Autodesk Inventor part; units mm, degrees
ref_plane "YZ Plane" through (0, 0, 0) normal (1, 0, 0) x (0, 1, 0)
ref_plane "XZ Plane" through (0, 0, 0) normal (0, 1, 0) x (-1, 0, 0)
ref_plane "XY Plane" through (0, 0, 0) normal (0, 0, 1) x (1, 0, 0)
sketch "Sketch1" plane through (0, 0, 0) normal (0, 0, 1) x (1, 0, 0)
  circle A0 centre (0, 0) radius 161.1083
  line L0 (4.75, 161.0382) -> (4.75, -161.0382)
  line L1 (-4.75, -161.0382) -> (-4.75, 161.0382)
  line L2 (0, 0) -> (0, 161.1083) construction
  line L3 (23.8125, 79.375) -> (23.8125, 47.625)
  line L4 (23.8125, 47.625) -> (51.3088, 63.5)
  line L5 (51.3088, 63.5) -> (23.8125, 79.375)
  line L6 (23.8125, 111.125) -> (23.8125, 79.375)
  line L7 (23.8125, 79.375) -> (51.3088, 95.25)
  line L8 (51.3088, 95.25) -> (23.8125, 111.125)
  line L9 (23.8125, 47.625) -> (23.8125, 15.875)
  line L10 (23.8125, 15.875) -> (51.3088, 31.75)
  line L11 (51.3088, 31.75) -> (23.8125, 47.625)
  line L12 (23.8125, 15.875) -> (23.8125, -15.875)
  line L13 (23.8125, -15.875) -> (51.3088, 0)
  line L14 (51.3088, 0) -> (23.8125, 15.875)
  line L15 (23.8125, -15.875) -> (23.8125, -47.625)
  line L16 (23.8125, -47.625) -> (51.3088, -31.75)
  line L17 (51.3088, -31.75) -> (23.8125, -15.875)
  line L18 (23.8125, -47.625) -> (23.8125, -79.375)
  line L19 (23.8125, -79.375) -> (51.3088, -63.5)
  line L20 (51.3088, -63.5) -> (23.8125, -47.625)
  line L21 (23.8125, -79.375) -> (23.8125, -111.125)
  line L22 (23.8125, -111.125) -> (51.3088, -95.25)
  line L23 (51.3088, -95.25) -> (23.8125, -79.375)
  line L24 (51.3088, 95.25) -> (78.8051, 79.375)
  line L25 (78.8051, 79.375) -> (51.3088, 63.5)
  line L26 (51.3088, 63.5) -> (78.8051, 47.625)
  line L27 (78.8051, 47.625) -> (51.3088, 31.75)
  line L28 (51.3088, 31.75) -> (78.8051, 15.875)
  line L29 (78.8051, 15.875) -> (51.3088, 0)
  line L30 (51.3088, 0) -> (78.8051, -15.875)
  line L31 (78.8051, -15.875) -> (51.3088, -31.75)
  line L32 (51.3088, -31.75) -> (78.8051, -47.625)
  line L33 (78.8051, -47.625) -> (51.3088, -63.5)
  line L34 (51.3088, -63.5) -> (78.8051, -79.375)
  line L35 (78.8051, -79.375) -> (51.3088, -95.25)
  line L36 (78.8051, -47.625) -> (106.3014, -31.75)
  line L37 (106.3014, -31.75) -> (78.8051, -15.875)
  line L38 (78.8051, -15.875) -> (106.3014, 0)
  line L39 (106.3014, 0) -> (78.8051, 15.875)
  line L40 (78.8051, 15.875) -> (106.3014, 31.75)
  line L41 (106.3014, 31.75) -> (78.8051, 47.625)
  line L42 (0, 0) -> (106.066, 106.066) construction
  point P0 (23.8125, 0)
  point P1 (78.8051, 79.375)
  dimension "d0" = 322.2165
  dimension "d2" = 9.5
  dimension "d3" = 4.75
  dimension "d4" = 31.75
  dimension "d5" = 31.75
  dimension "d6" = 31.75
  dimension "d7" = 31.75
  dimension "d8" = 31.75
  dimension "d9" = 31.75
  dimension "d10" = 31.75
  dimension "d27" = 23.8125
  dimension "d28" = 150
  dimension "d29" = 45
extrude "Extrusion1" add sketch "Sketch1" along normal blind 28.575 contours A0 L0 | L0 A0 L1 | L1 A0 | L5 L4 L3 | L7 L24 L25 L5 | L6 L8 L7 | L11 L10 L9 | L4 L26 L27 L11 | L14 L13 L12 | L10 L28 L29 L14 | L27 L41 L40 L28 | L17 L16 L15 | L13 L30 L31 L17 | L29 L39 L38 L30 | L20 L19 L18 | L16 L32 L33 L20 | L31 L37 L36 L32 | L23 L22 L21 | L19 L34 L35 L23
hole "Hole2" at (23.8125, 47.625, 0) at (51.3088, 63.5, 0) at (23.8125, 111.125, 0) at (23.8125, 79.375, 0) at (51.3088, 95.25, 0) at (51.3088, 31.75, 0) at (23.8125, 15.875, 0) at (23.8125, -15.875, 0) at (51.3088, 0, 0) at (23.8125, -47.625, 0) at (51.3088, -31.75, 0) at (23.8125, -79.375, 0) at (51.3088, -63.5, 0) at (23.8125, -111.125, 0) at (51.3088, -95.25, 0) at (78.8051, 79.375, 0) at (78.8051, 47.625, 0) at (78.8051, 15.875, 0) at (78.8051, -15.875, 0) at (78.8051, -47.625, 0) at (78.8051, -79.375, 0) at (106.3014, -31.75, 0) at (106.3014, 31.75, 0) direction (0, 0, 1) diameter 25.4 end up to surface
mirror "Mirror1" about plane through (0, 0, 0) normal (1, 0, 0) of "Hole2"
hole "Hole3" at (106.066, 106.066, 0) direction (0, 0, 1) diameter 9.5 end up to surface
pattern_circular "Circular Pattern1" count 4 over 360 about axis through (0, 0, 0) along (0, 0, 1) of "Hole3"
properties part number "Tube Sheet" material "Titanium"
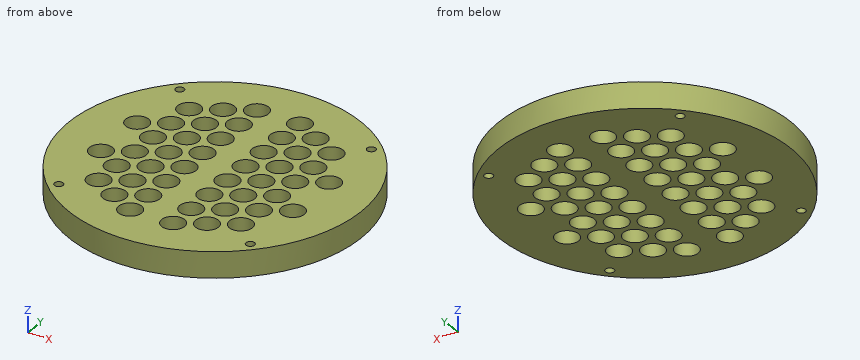
Source: CAD feature listing. Evaluate the final solid. Frame: model axes, mm. Give positions to 0.01 mm unless a question says otherwise; leave off trailing zeros. Loops run counter-clockwise (first coordinate to the right, second up) from the corner with the lowest first, then second, coordinate; pieces in that order, holes last. Notation, with made-up numbers: M 60.5,20.5 L 88.5,20.5 A35 cw 88.5,59.5 Z; hole C 82.25,26 d11. An arc over 180 degrees is marked long. Put each result on its own line as item: value.
Q1. Section C-C (x = 131.5). Return the cut outline in (y, z) (3 decimals).
Response values:
outline: M -93.079,0 L 93.079,0 L 93.079,28.575 L -93.079,28.575 Z
Q2. Pin query (flat end, axial travel): P1, Ø8, axis at y = -110, z = 20.5, coming from the -X side; P2, Ø4, axis at x = 81, z = 13.5, coming from the +Y side; P3, Ø6, axis at x = -16.5, z = 12.5, coming from the -Y side; P4, Ø3, axis at x = 81.5, y = 122, coming from the -Z side. Return the tip coordinate at first contact, or that it passes through.
Response values:
P1: stops at x = -121.33
P2: stops at y = 140.41
P3: stops at y = -160.54
P4: stops at z = 0
Q3. Line query: probe 1 along X at (y, z) = (93, 25); probe 2 along Y at (x, z) = (98, 24.5); probe 3 along X at (y, z) = (95.25, 18). Output: solid intervals per line, ascending. Write a range as [from, to].
Response values:
probe 1: x = [-131.56, -63.81], [-38.81, 38.81], [63.81, 131.56]
probe 2: y = [-127.87, -41.36], [-22.14, 22.14], [41.36, 127.87]
probe 3: x = [-129.94, -64.01], [-38.61, 38.61], [64.01, 129.94]
Q4. Section B-B (z = 23). Count the separate pieces of the cut face and the enclosed holes in it, and give its area (3 significant figures).
Response values:
separate pieces: 1
enclosed holes: 50
area: 58,000 mm²
Q5. Section A-A (x = -85). Return the cut outline in (y, z) (3 decimals).
Response values:
outline: M -136.861,0 L -90.462,0 L -90.462,28.575 L -136.861,28.575 Z; M -68.288,0 L -58.712,0 L -58.712,28.575 L -68.288,28.575 Z; M -36.538,0 L -26.962,0 L -26.962,28.575 L -36.538,28.575 Z; M -4.788,0 L 4.788,0 L 4.788,28.575 L -4.788,28.575 Z; M 26.962,0 L 36.538,0 L 36.538,28.575 L 26.962,28.575 Z; M 58.712,0 L 68.288,0 L 68.288,28.575 L 58.712,28.575 Z; M 90.462,0 L 136.861,0 L 136.861,28.575 L 90.462,28.575 Z
